The listing builds one solid part. Answer for the finished solid, in the listing's coordinates (mm). A direction names the side the tool comes from. Round coordinates to 2 decimals unless told otherwise and drop trailing zeros. Loops run counter-clockwise (first coordinate to the right, second up) from the corner with the lowest first, then second, coordinate; pieces in that order, holes last. Notation, with made-up numbers: (89, 11) -> (147, 11) arc R3 cw to (147, 15) -> close; hole circle Ø6 at (45.25, 27.25). An arc over 180 degrees is marked (long way). One line per question, with ' | ' between items.
Autodesk Inventor part; units mm, degrees
ref_plane "YZ Plane" through (0, 0, 0) normal (1, 0, 0) x (0, 1, 0)
ref_plane "XZ Plane" through (0, 0, 0) normal (0, 1, 0) x (-1, 0, 0)
ref_plane "XY Plane" through (0, 0, 0) normal (0, 0, 1) x (1, 0, 0)
sketch "Sketch1" plane through (0, 0, 0) normal (0, 0, 1) x (1, 0, 0)
  line L0 (0, 0) -> (455.7, 0)
  line L1 (455.7, 0) -> (455.7, 335)
  line L2 (455.7, 335) -> (0, 335)
  line L3 (0, 335) -> (0, 0)
  dimension "d0" = 455.7
  dimension "d1" = 335
extrude "Extrusion1" add sketch "Sketch1" along normal blind 4.7625
sketch "Sketch3" plane through (0, 0, 4.7625) normal (0, 0, 1) x (1, 0, 0)
  line L0 (0, 0) -> (455.7, 0)
  line L1 (0, 335) -> (0, 0)
  line L2 (0, 61) -> (6, 61)
  line L3 (6, 61) -> (6, 20)
  line L4 (455.7, 335) -> (0, 335)
  line L5 (0, 244) -> (6, 244)
  line L6 (6, 244) -> (6, 285)
  line L7 (6, 285) -> (0, 285)
  line L8 (6, 20) -> (0, 20)
  dimension "d11" = 41
  dimension "d12" = 6
  dimension "d15" = 41
  dimension "d16" = 6
  dimension "d27" = 50
  dimension "d28" = 20
extrude "Extrusion3" cut sketch "Sketch3" against normal up to next
sketch "Sketch4" plane through (0, 0, 0) normal (0, 0, -1) x (-1, 0, 0)
  line L0 (-6, 244) -> (-6, 285)
  line L1 (-455.7, 335) -> (0, 335)
  line L2 (0, 0) -> (-455.7, 0)
  line L3 (-6, 20) -> (-6, 61)
  line L4 (-6, 244) -> (-20.5, 244)
  line L5 (-20.5, 244) -> (-20.5, 285)
  line L6 (-6, 61) -> (-20.5, 61)
  line L7 (-20.5, 61) -> (-20.5, 20)
  line L8 (-6, 285) -> (-20.5, 285)
  line L9 (-20.5, 20) -> (-6, 20)
  point P0 (-6, 335)
  point P1 (-6, 0)
  dimension "d17" = 14.5
  dimension "d18" = 14.5
extrude "Extrusion4" cut sketch "Sketch4" against normal blind 2
sketch "Sketch5" plane through (0, 0, 4.7625) normal (0, 0, 1) x (1, 0, 0)
  line L0 (455.7, 0) -> (455.7, 335)
  line L1 (455.7, 335) -> (0, 335)
  circle A0 centre (411.7, 217.5) radius 2.5
  circle A1 centre (411.7, 117.5) radius 2.5
  point P0 (6, 335)
  dimension "d21" = 5
  dimension "d22" = 100
  dimension "d23" = 117.5
  dimension "d24" = 44
extrude "Extrusion5" cut sketch "Sketch5" against normal up to next
sketch "Sketch6" plane through (0, 0, 2) normal (0, 0, -1) x (-1, 0, 0)
  line L0 (-20.5, 285) -> (-6, 285)
  line L1 (-6, 244) -> (-20.5, 244)
  line L2 (-6, 61) -> (-6, 20)
  line L3 (-20.5, 61) -> (-6, 61)
  line L4 (-20.5, 20) -> (-20.5, 61)
  line L5 (-6, 20) -> (-20.5, 20)
  circle A0 centre (-12, 277) radius 2.75
  circle A1 centre (-12, 252) radius 2.75
  circle A2 centre (-12, 53) radius 2.75
  circle A3 centre (-12, 28) radius 2.75
  point P0 (0, 0)
  dimension "d29" = 5.5
  dimension "d30" = 5.5
  dimension "d31" = 5.5
  dimension "d32" = 5.5
  dimension "d34" = 8
  dimension "d35" = 8
  dimension "d36" = 8.5
  dimension "d37" = 8
  dimension "d38" = 8
extrude "Extrusion6" cut sketch "Sketch6" against normal up to next contours A0 | A1 | A2 | A3
properties part number "EnclosureDoorFront" material "Polycarbonate, Clear"
Q1. For faces 1 (the face through (225, 170, 0)), 2 (the face through (13, 265, 2)), determine the directions among +Z, -Z, +X, -X, +Y, -Y from which every point of the face is accessible in a straight line to the end or side of a thin tool.
Numbers:
face 1: -Z, +X, -X, +Y, -Y | face 2: -Z, -X
Q2. Find the intervals of material crossed by line 1 (Y direction, x = 411.7, z = 2.6); line 2 (Y direction, x = 12, z = 3.2); line 3 (X direction, y = 217.5, z = 1.3), in increasing order. Write a range as from..to.
Numbers:
line 1: 0..115, 120..215, 220..335 | line 2: 0..25.25, 30.75..50.25, 55.75..249.25, 254.75..274.25, 279.75..335 | line 3: 0..409.2, 414.2..455.7
Q3. Given pin 1 Ø2 at (y, z) = (272.5, 0.5) entering from -X; pin 2 Ø3.5 at (x, y) = (12, 28) entering from +Z; pin 3 Ø1.4 at (y, z) = (32, 3.5) entering from -X; pin 4 Ø7 at (x, y) = (12, 53) entering from -Z, each flat-ended and moving along its own axis, determine where each tip first touches the part or whether it passes through.
Numbers:
pin 1: x = 20.5 | pin 2: through | pin 3: x = 6 | pin 4: z = 2
Q4. A cutting plane is placed at A-A on y = 36. Give the vertices of the cut face in (x, z), plus the area to 3 significant figures.
Numbers:
outline: (6, 2) -> (20.5, 2) -> (20.5, 0) -> (455.7, 0) -> (455.7, 4.76) -> (6, 4.76) -> close | area: 2,110 mm^2
